```python
from build123d import *

# Parameters (mm, degrees)
F1_DEPTH = 80.518
F3_DEPTH = 9.398
F4_W     = 1.524
F4_H     = 1.524
F5_DEPTH = 80.519
F7_DEPTH = 27.178
F9_DEPTH = 14.478


with BuildPart() as f1:
    # F0 (on Front) → F1 (new body)
    with BuildSketch(Plane.XZ):
        with BuildLine():
            ThreePointArc((40.259, 11.811), (38.027154, 17.199154), (32.639, 19.431))
            Line((32.639, 19.431), (-32.639, 19.431))
            ThreePointArc((-32.639, 19.431), (-38.027154, 17.199154), (-40.259, 11.811))
            Line((-40.259, 11.811), (-40.259, -11.811))
            ThreePointArc((-40.259, -11.811), (-38.027154, -17.199154), (-32.639, -19.431))
            Line((-32.639, -19.431), (32.639, -19.431))
            ThreePointArc((32.639, -19.431), (38.027154, -17.199154), (40.259, -11.811))
            Line((40.259, -11.811), (40.259, 11.811))
        make_face()
    extrude(amount=F1_DEPTH)

    # F2 (on face) → F3 (cut)
    with BuildSketch(Plane.XZ.offset(80.518)):
        with BuildLine():
            ThreePointArc((30.48, 6.731), (28.992102, 10.323102), (25.4, 11.811))
            Line((25.4, 11.811), (-25.4, 11.811))
            ThreePointArc((-25.4, 11.811), (-28.992102, 10.323102), (-30.48, 6.731))
            Line((-30.48, 6.731), (-30.48, -6.731))
            ThreePointArc((-30.48, -6.731), (-28.992102, -10.323102), (-25.4, -11.811))
            Line((-25.4, -11.811), (25.4, -11.811))
            ThreePointArc((25.4, -11.811), (28.992102, -10.323102), (30.48, -6.731))
            Line((30.48, -6.731), (30.48, 6.731))
        make_face()
    extrude(amount=-F3_DEPTH, mode=Mode.SUBTRACT)

    # F4 (on face) → F5 (cut, through all)
    with BuildSketch(Plane.XZ.offset(80.518)):
        with Locations((-39.497, 11.049)):
            Rectangle(F4_W, F4_H)
        with Locations((39.497, 11.049)):
            Rectangle(F4_W, F4_H)
    extrude(amount=-F5_DEPTH, mode=Mode.SUBTRACT)

    # F6 (on face) → F7 (cut)
    with BuildSketch(Plane.XY.offset(19.431)):
        with BuildLine():
            Line((19.939, -20.066), (-20.193, -20.066))
            ThreePointArc((-20.193, -20.066), (-23.785102, -21.553898), (-25.273, -25.146))
            Line((-25.273, -25.146), (-25.273, -55.372))
            ThreePointArc((-25.273, -55.372), (-23.785102, -58.964102), (-20.193, -60.452))
            Line((-20.193, -60.452), (19.939, -60.452))
            ThreePointArc((19.939, -60.452), (23.531102, -58.964102), (25.019, -55.372))
            Line((25.019, -55.372), (25.019, -25.146))
            ThreePointArc((25.019, -25.146), (23.531102, -21.553898), (19.939, -20.066))
        make_face()
    extrude(amount=-F7_DEPTH, mode=Mode.SUBTRACT)

    # F8 (on face) → F9 (cut)
    with BuildSketch(Plane(origin=(0, 0, 0), x_dir=(-1, 0, 0), z_dir=(0, 1, 0))):
        with BuildLine():
            ThreePointArc((31.75, 7.62), (30.262102, 11.212102), (26.67, 12.7))
            Line((26.67, 12.7), (-26.67, 12.7))
            ThreePointArc((-26.67, 12.7), (-30.262102, 11.212102), (-31.75, 7.62))
            Line((-31.75, 7.62), (-31.75, -7.62))
            ThreePointArc((-31.75, -7.62), (-30.262102, -11.212102), (-26.67, -12.7))
            Line((-26.67, -12.7), (26.67, -12.7))
            ThreePointArc((26.67, -12.7), (30.262102, -11.212102), (31.75, -7.62))
            Line((31.75, -7.62), (31.75, 7.62))
        make_face()
    extrude(amount=-F9_DEPTH, mode=Mode.SUBTRACT)


solid = f1.part
```
The model under review builds one solid part; all positions refer to its coordinate system, in mm. A direction names the side the tool comes from. Round coordinates to 2 decimals unless told otherwise and drop trailing zeros. Write each loop counter-clockwise with the first axis right and the second up, starting at its lowest first coordinate (ties: lowest second). Pieces come first, ordered by that corner, then holes. Notation, with made-up numbers: (-13.5, 29) - (35.5, 29) arc R14 cw to (35.5, 35) - close; hole circle Ø5 at (29, -25). An arc over 180 degrees is marked (long way). Use one line per item in the form item = value.
Q1. Consider section C-C (y = -66.5). State the section outline as (x, z) points (3 decimals), and give its area (3 significant figures).
Answer key:
outline = (-40.259, -11.811) arc R7.62 ccw to (-32.639, -19.431) - (32.639, -19.431) arc R7.62 ccw to (40.259, -11.811) - (40.259, 10.287) - (38.735, 10.287) - (38.735, 11.811) - (40.259, 11.811) arc R7.62 ccw to (32.639, 19.431) - (-32.639, 19.431) arc R7.62 ccw to (-40.259, 11.811) - (-38.735, 11.811) - (-38.735, 10.287) - (-40.259, 10.287) - close
area = 3,070 mm2
Q2. Tool access review of faces 1 (the flat face through (-25.273, -40, 6)), 2 (the flat face through (-1, 0, 13)), 3 (the cylindrical face through (-30.222, -7.138, -11.251)), 4 (the cylindrical face through (-29.031, -75.885, -10.283)): name each direction out of +Z, -Z, +X, -X, +Y, -Y from which nothing blocks a thin tool from reaching the whole face with its end or side.
Answer key:
face_1 = +Z
face_2 = +Z, -Z, +X, -X, +Y
face_3 = +Y
face_4 = -Y
Q3. Consider section A-A (z = -3). State the section outline as (x, y) points.
Answer key:
outline = (-40.26, -80.52) - (-30.48, -80.52) - (-30.48, -71.12) - (30.48, -71.12) - (30.48, -80.52) - (40.26, -80.52) - (40.26, 0) - (31.75, 0) - (31.75, -14.48) - (-31.75, -14.48) - (-31.75, 0) - (-40.26, 0) - close; hole (-25.27, -55.37) arc R5.08 ccw to (-20.19, -60.45) - (19.94, -60.45) arc R5.08 ccw to (25.02, -55.37) - (25.02, -25.15) arc R5.08 ccw to (19.94, -20.07) - (-20.19, -20.07) arc R5.08 ccw to (-25.27, -25.15) - close
Q4. Insertion check: pin 1 Ø12.5 at (x, z) = (-0.5, 1.5) entering from +Y; pin 2 Ø8 at (x, z) = (9, 6) entering from -Y; pin 3 Ø1.7 at (x, y) = (39.5, -55.5) entering from -Z; pin 4 Ø5 at (x, z) = (-7, -12.5) entering from +Y. Each pin has a flat end and moves straight along its axis. Give the tip position at first contact, or say it passes through.
Answer key:
pin_1 = -14.48
pin_2 = -71.12
pin_3 = -16.49
pin_4 = 0
Q5. Draft analysis for pull direction X (two halves, no side actions). For faces 5 (the flat face through (-40.259, -40, -1)), 6 (the cylindrical face through (37.968, -39.695, -17.258)), 7 (the flat face through (0, -40, -7.747)), state which applies: +X half, -X half, draft (parallel to the pull), parting line (faces both ways), or undercut.
Answer key:
face_5 = -X half
face_6 = +X half
face_7 = undercut
Q6. For line 1 (X direction, y = -2.5, z = -3.5); line 2 (Y direction, x = -18.5, z = 5); line 3 (X direction, y = -46.5, z = 3.5), list the stretches that pass through material, from the lowest coordinate up. Write a range as [from, to].
Answer key:
line_1 = [-40.26, -31.75], [31.75, 40.26]
line_2 = [-71.12, -60.45], [-20.07, -14.48]
line_3 = [-40.26, -25.27], [25.02, 40.26]
Q7. Consider section D-D (z = 14). State the section outline as (x, y) points.
Answer key:
outline = (-39.94, -80.52) - (39.94, -80.52) - (39.94, 0) - (-39.94, 0) - close; hole (-25.27, -55.37) arc R5.08 ccw to (-20.19, -60.45) - (19.94, -60.45) arc R5.08 ccw to (25.02, -55.37) - (25.02, -25.15) arc R5.08 ccw to (19.94, -20.07) - (-20.19, -20.07) arc R5.08 ccw to (-25.27, -25.15) - close
Q8. Consider section B-B (x = 12.5). State the section outline as (y, z) points.
Answer key:
outline = (-80.52, -19.43) - (0, -19.43) - (0, -12.7) - (-14.48, -12.7) - (-14.48, 12.7) - (0, 12.7) - (0, 19.43) - (-20.07, 19.43) - (-20.07, -7.75) - (-60.45, -7.75) - (-60.45, 19.43) - (-80.52, 19.43) - (-80.52, 11.81) - (-71.12, 11.81) - (-71.12, -11.81) - (-80.52, -11.81) - close
